Geometry: see drawing. Coordinates: mm, zero at the bounding-box minimum. A direction names the side the tool comes from. Give positions to 0.01 mm unless a question says otherwise; leave off trailing zeros. Order: outer loops, then holes, each group sorted by start corner. A loop starts at its lowest first (then second) coordinate and runs counter-clockwise, first axis right, second up. Notation, with made-up numbers: M 47,-32.5 L 105,-32.5 A16 cw 105,-1.5 Z; hole C -33.75,46.25 d11. An arc over 180 degrees is marked long. Write item = value, one per line. Start each with the question number.
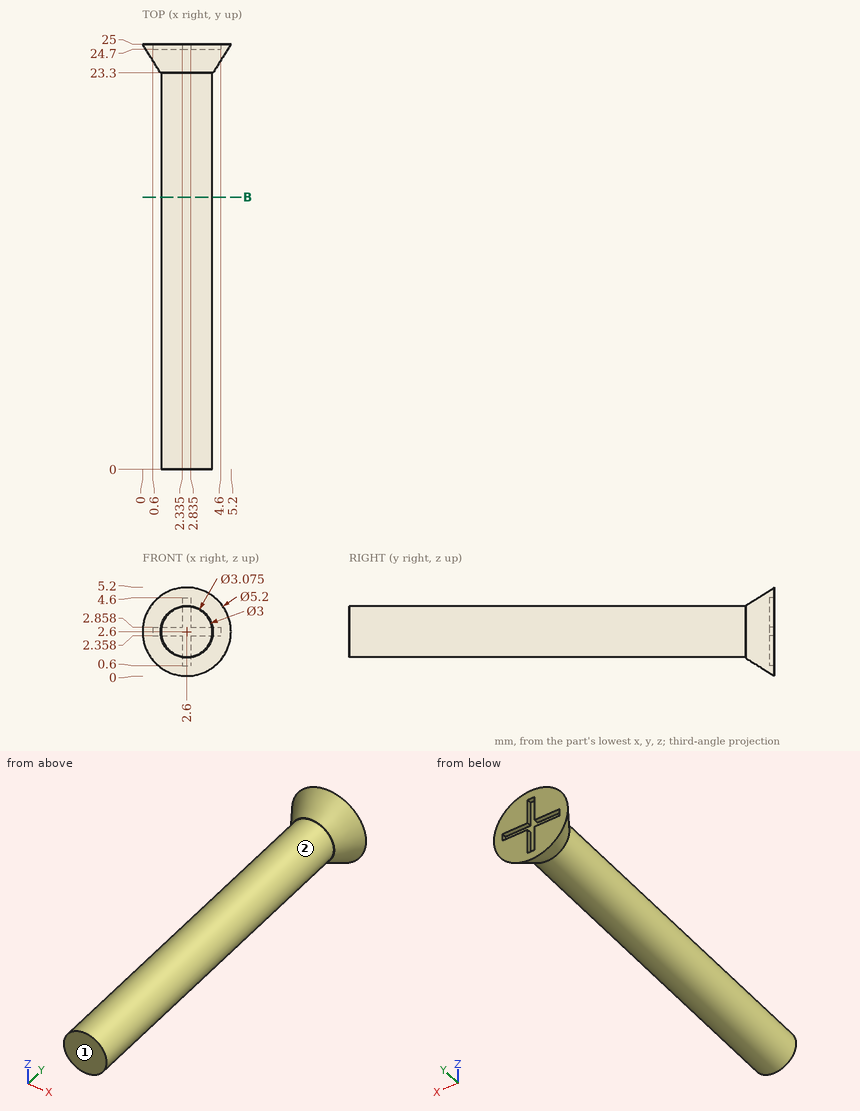
1) Cut plane B-B (y = 16). Return loops of the section in (x, z).
2) Ray query, L1, parallel to X at y = 20.5, z = 2.5; L2, parallel to Y at x = 2.3, z = 2.75; L3, parallel to Z at x = 1.9, y = 18 (1 decimal). Return the intervals inside material, ascending.
3) Access query for the marked faces 1 and 2. Directions: +Z, -Z, +X, -X, +Y, -Y. A direction counts if a zero-diameter tool reaches every point of the face in a straight line with its end or side. Return the directions, or none.
4) Pin query (flat end, axial travel): pin 1 Ø3 at (x, y) = (0.5, 13) entering from +Z (1 decimal); pin 2 Ø1 at (y, z) = (6.5, 2) entering from +X. Return the tip coordinate at first contact, or that it passes through.
Reply:
q1.outline = C 2.6,2.6 d3
q2.L1 = 1.1 to 4.1
q2.L2 = 0 to 24.7
q2.L3 = 1.3 to 3.9
q3.face_1 = +Z, -Z, +X, -X, -Y
q3.face_2 = -Y
q4.pin_1 = 4
q4.pin_2 = 4.1
